Input: part model. Units: mm. Frame: model coordinates. Coordinates: 2 decimals unless noted, no trailing zeros. Write each loop counter-clockwise with the first axis right and the second up, starting at its lowest first coordinate (ties: lowest second). Pieces come first, ordered by that corner, then holes. Notation, with made-up numbers: (51, 75) - (84, 75) arc R22 ccw to (84, 85) - close; hole circle Ø2 at (75, 53). An arc over 180 degrees is marked (long way). Use a Markdown table: item, result. Add a question column.
Q1. Section query A-A (z = -26.1). Return the cut outline in (x, y).
Q2. Material intervals for probe 1 along Z at (x, y) = (22.25, 0.65); probe 2 along Z at (x, y) = (10.5, 0.9); probe 3 along X at (y, z) = (1.15, -26.1), sorted ascending. Write a range as from..to.
Q3. Section query B-B (x = 14.5). Return the cut outline in (y, z).
Q4. Section query D-D (y = 0.8). Return the cut outline in (x, z), then the cut area to 3 significant figures.
Q5. Section query C-C (z = -8). Return the cut outline in (x, y), then the cut area to 3 significant figures.
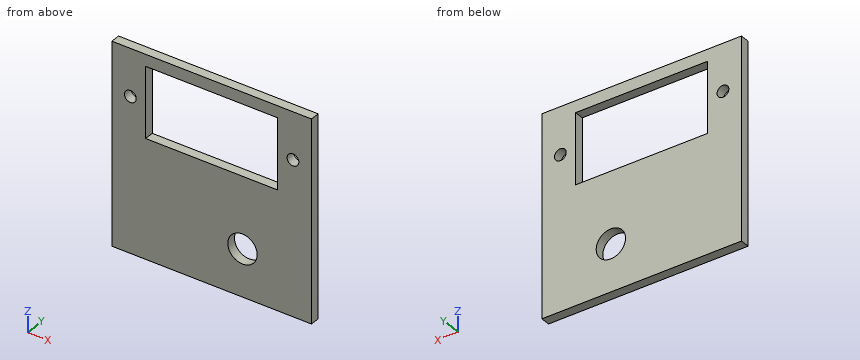
Autodesk Inventor part; units mm, degrees
ref_plane "YZ Plane" through (0, 0, 0) normal (1, 0, 0) x (0, 1, 0)
ref_plane "XZ Plane" through (0, 0, 0) normal (0, 1, 0) x (-1, 0, 0)
ref_plane "XY Plane" through (0, 0, 0) normal (0, 0, 1) x (1, 0, 0)
sketch "Szkic1" plane through (0, 0, 0) normal (0, 1, 0) x (-1, 0, 0)
  line L0 (0, 0) -> (-34, 0)
  line L1 (-34, 0) -> (-34, -34.1)
  line L2 (-34, -34.1) -> (0, -34.1)
  line L3 (0, -34.1) -> (0, 0)
  line L4 (-5.75, -2) -> (-28.25, -2)
  line L5 (-28.25, -2) -> (-28.25, -14)
  line L6 (-28.25, -14) -> (-5.75, -14)
  line L7 (-5.75, -14) -> (-5.75, -2)
  circle A0 centre (-3.15, -8) radius 1
  circle A1 centre (-30.85, -8) radius 1
  dimension "d0" = 34
  dimension "d1" = 34.1
  dimension "d2" = 22.5
  dimension "d3" = 12
  dimension "d4" = 2
  dimension "d5" = 5.75
  dimension "d6" = 2
  dimension "d7" = 2.6
  dimension "d8" = 2
  dimension "d9" = 2.6
  dimension "d12" = 6
  dimension "d13" = 6
extrude "Wyciągnięcie proste1" add sketch "Szkic1" along normal blind 1.6
sketch "Szkic2" plane through (0, 1.6, 0) normal (0, 1, 0) x (1, 0, 0)
  circle A0 centre (22.25, 26.1) radius 2.5
  line L0 (34, 0) -> (34, 34.1)
  line L1 (34, 34.1) -> (0, 34.1)
  point P0 (0, 0)
  dimension "d14" = 5
  dimension "d15" = 11.75
  dimension "d16" = 8
extrude "Wyciągnięcie proste2" cut sketch "Szkic2" against normal blind 1.6
equation "\"d5\" = -0.5 * d2 + 0.5 * d0"
equation "\"d12\" = 0.5 * d3"
equation "\"d13\" = d12"
properties part number "mocowanie ostatniego serwa"
Values follow:
| question | item | result |
|---|---|---|
| 1 | outline | (0, 0) - (19.75, 0) - (19.75, 1.6) - (0, 1.6) - close; (24.75, 0) - (34, 0) - (34, 1.6) - (24.75, 1.6) - close |
| 2 | probe 1 | -34.1..-28.6, -23.6..-14, -2..0 |
| 2 | probe 2 | -34.1..-14, -2..0 |
| 2 | probe 3 | 0..19.75, 24.75..34 |
| 3 | outline | (0, -34.1) - (1.6, -34.1) - (1.6, -14) - (0, -14) - close; (0, -2) - (1.6, -2) - (1.6, 0) - (0, 0) - close |
| 4 | outline | (0, -34.1) - (34, -34.1) - (34, 0) - (0, 0) - close; hole circle Ø2 at (3.15, -8); hole (5.75, -14) - (28.25, -14) - (28.25, -2) - (5.75, -2) - close; hole circle Ø5 at (22.25, -26.1); hole circle Ø2 at (30.85, -8) |
| 4 | area | 863 mm2 |
| 5 | outline | (0, 0) - (2.15, 0) - (2.15, 1.6) - (0, 1.6) - close; (4.15, 0) - (5.75, 0) - (5.75, 1.6) - (4.15, 1.6) - close; (28.25, 0) - (29.85, 0) - (29.85, 1.6) - (28.25, 1.6) - close; (31.85, 0) - (34, 0) - (34, 1.6) - (31.85, 1.6) - close |
| 5 | area | 12.0 mm2 |
